Source: CAD feature listing. Evaluate the final solid. Frame: model axes, mm. Give positions to 0.01 mm unless a question says otherwise; leave off trailing zeros. Loops run counter-clockwise (first coordinate to the right, second up) from the corner with the lowest first, then second, coordinate; pieces in that order, holes last. Notation, with made-up numbers: M 35.25,-15 L 52.25,-15 A18 ccw 52.25,2 Z; hole C 54,6.25 d9. An arc over 180 degrees is marked long. Answer in a Markdown table with one row per item.
```python
from build123d import *

# Parameters (mm, degrees)
ENL_V_MAT_EXTRU_2_DEPTH = 0.72
CONG_4_R                = 0.24


with BuildPart() as part:
    # Esquisse1 → Révolution1 (revolve)
    with BuildSketch(Plane(origin=(0, 0, 0), x_dir=(0, 0, -1), z_dir=(1, 0, 0))):
        with BuildLine():
            Line((9.12, 0), (0, 0))
            Line((0, 0), (0, 2.4))
            ThreePointArc((0, 2.4), (0.070294373, 2.569705627), (0.24, 2.64))
            Line((0.24, 2.64), (1.92, 2.64))
            Line((1.92, 2.64), (1.92, 2.11316162))
            Line((1.92, 2.11316162), (9.12, 0.318))
            Line((9.12, 0.318), (9.12, 0))
        make_face()
    revolve(axis=Axis((0, 0, -9.12), (0, 0, 1)))

    # Esquisse3 → Enlèv. mat.-Extru.2 (cut)
    with BuildSketch(Plane.XY):
        Polygon((0.32, 1.578), (-0.32, 1.578), (-0.32, 0.318), (-1.584, 0.318), (-1.584, -0.318), (-0.32, -0.318), (-0.32, -1.578), (0.32, -1.578), (0.32, -0.318), (1.584, -0.318), (1.584, 0.318), (0.32, 0.318), align=None)
    extrude(amount=-ENL_V_MAT_EXTRU_2_DEPTH, mode=Mode.SUBTRACT)

    # Congé4
    cong_4_edges = [part.edges().sort_by_distance(p)[0] for p in [
        (0, -1.578, -0.72),
        (-1.584, 0, -0.72),
        (0, 1.578, -0.72),
        (1.584, 0, -0.72),
    ]]
    fillet(cong_4_edges, radius=CONG_4_R)


solid = part.part
```
Q1. Section query D-D (z = -8). Output: boundary loops of the cut face in (x, y).
Values follow:
| item | result |
|---|---|
| outline | C 0,0 d1.19 |
Q2. Ray query, probe 1 along Z at (x, y) = (0.15, 0); probe 2 along Z at (x, y) = (0.6, 2.1); probe 3 along Y at (x, z) = (0.6, -0.5). Return the intervals inside material, ascending. Write a range as from..to.
Values follow:
| item | result |
|---|---|
| probe 1 | -9.12..-0.72 |
| probe 2 | -1.92..0 |
| probe 3 | -2.57..-0.32, 0.32..2.57 |
Q3. Contact query for flat-ended pins moving along their axis: pin 1 Ø2 at (x, y) = (1, 0) entering from +Z; pin 2 Ø0.6 at (x, z) = (1, -0.5) entering from +Y; pin 3 Ø0.6 at (x, z) = (1, 0) entering from -Y; pin 4 Ø1.5 at (y, z) = (0.5, -4.5) entering from -X. Output: stop coordinate, or through.
Values follow:
| item | result |
|---|---|
| pin 1 | z = 0 |
| pin 2 | y = 2.55 |
| pin 3 | y = -2.52 |
| pin 4 | x = -1.63 |
Q4. Section query A-A (x = 0). Output: boundary loops of the cut face in (y, z).
Values follow:
| item | result |
|---|---|
| outline | M -2.64,-1.92 L -2.11,-1.92 L -0.32,-9.12 L 0.32,-9.12 L 2.11,-1.92 L 2.64,-1.92 L 2.64,-0.24 A0.24 ccw 2.4,0 L 1.58,0 L 1.58,-0.48 A0.24 cw 1.34,-0.72 L -1.34,-0.72 A0.24 cw -1.58,-0.48 L -1.58,0 L -2.4,0 A0.24 ccw -2.64,-0.24 Z |
Q5. Mould query, pull axis Y, two halves, no side actions, for faces 1 (the flat face through (0.5, -0.5, 0)), 2 (the flat face through (0, 0, -0.72)), 3 (the cylindrical face through (2.577, -0.572, -1.092)). Classes: +Y half, -Y half, draft (parallel to the pull), parting line (faces both ways), or undercut.
Values follow:
| item | result |
|---|---|
| face 1 | draft |
| face 2 | undercut |
| face 3 | parting line |
Q6. Section query C-C (z = -3.5). Output: boundary loops of the cut face in (x, y).
Values follow:
| item | result |
|---|---|
| outline | C 0,0 d3.44 |
